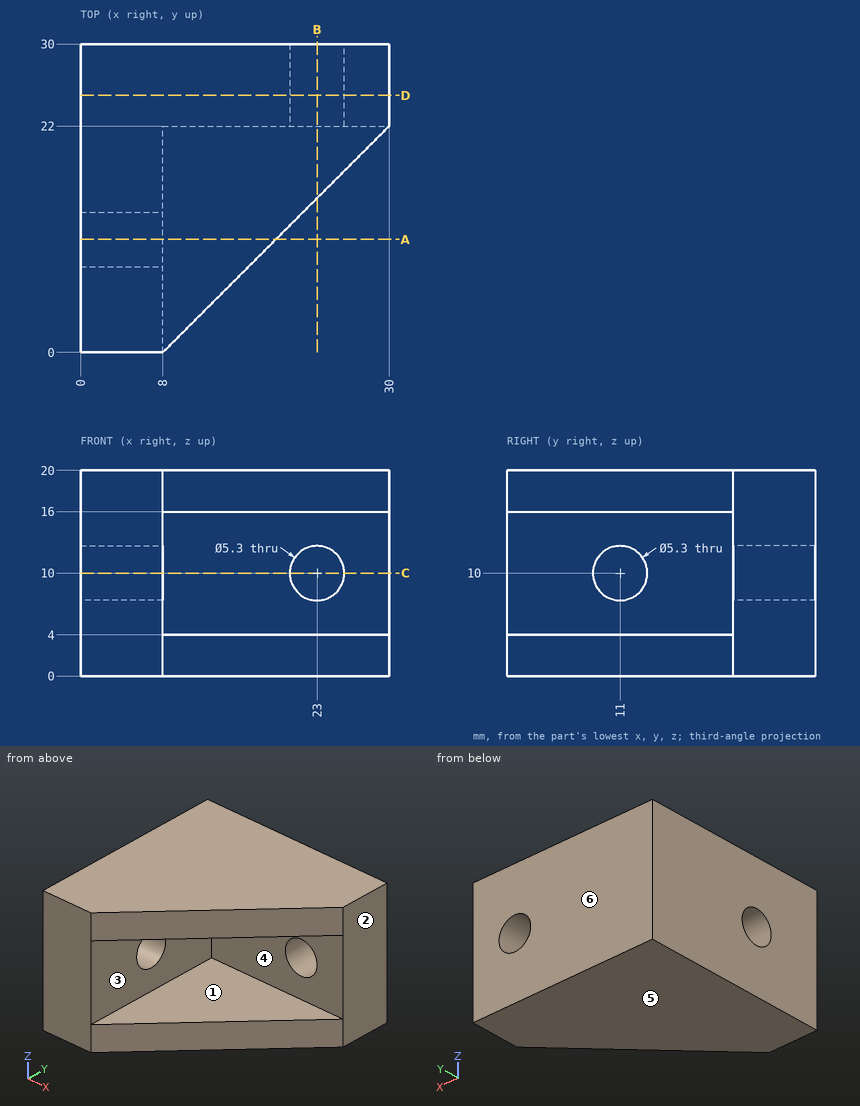
Answer from the drawing. Dimensions are ordinates in mm from the lowest x, y and z of the part. A direction names the side the tool comes from. Round coordinates to 2 decimals unless told otherwise and drop trailing zeros. Write each loop counter-clockwise with the first axis right and the second up, starting at its lowest first coordinate (ties: lowest second). Pieces come first, ordered by that corner, then holes. Notation, with made-up numbers: (39, 57) -> (81, 57) arc R18 cw to (81, 79) -> close; hole circle Ø5 at (18.25, -39). An arc over 180 degrees is marked (long way). Answer in a Markdown table with one row per item. Add a question column.
1) Given P1, Ø6, axis at y = 12, z = 7.5, coming from the -X side; P2, Ø5, axis at x = 23, z = 10, coming from the -Y side; P3, Ø1.5, axis at x = 11, z = 17, coming from the -Y side; P4, Ø1, axis at x = 11, z = 11, coming from the -Y side, each flat-ended and moving along its own axis, determine where each tip first touches the part or whether it passes through.
2) Determine the mould class of the marked faces 3, 4, 5 and 6 for opening direction Z: pulls with the +Z half, pulls with the -Z half, needs draft (parallel to the pull), parting line crosses it, or undercut.
3) Find section D-D, the plane y = 25. Determine the outline of the cut face in (x, z), and give its area (3 significant figures).
4) Find section B-B, the plane x = 23. Determine the outline of the cut face in (y, z), and give its area (3 significant figures).
5) Find section A-A, the plane y = 11. Determine the outline of the cut face in (x, z).
6) Consider line 1 (Z direction, x = 16.5, y = 12.5); line 2 (Z direction, x = 23, y = 24); line 3 (Y direction, x = 5.75, z = 10). Determine where each line is inside the solid, lowest interval first.
7) Find section C-C, the plane z = 10. Determine the outline of the cut face in (x, y).
8) Which of the six approach directions +Z, -Z, +X, -X, +Y, -Y give full straight-line access (tool end or side, diameter ignored) to the marked faces 1 and 2?
Findings below:
| question | item | result |
|---|---|---|
| 1 | P1 | x = 0 |
| 1 | P2 | through |
| 1 | P3 | y = 2.25 |
| 1 | P4 | y = 22 |
| 2 | face 3 | undercut |
| 2 | face 4 | undercut |
| 2 | face 5 | pulls with the -Z half |
| 2 | face 6 | needs draft |
| 3 | outline | (0, 0) -> (30, 0) -> (30, 20) -> (0, 20) -> close; hole circle Ø5.3 at (23, 10) |
| 3 | area | 578 mm² |
| 4 | outline | (15, 0) -> (30, 0) -> (30, 7.35) -> (22, 7.35) -> (22, 4) -> (15, 4) -> close; (15, 16) -> (22, 16) -> (22, 12.65) -> (30, 12.65) -> (30, 20) -> (15, 20) -> close |
| 4 | area | 174 mm² |
| 5 | outline | (0, 0) -> (19, 0) -> (19, 4) -> (8, 4) -> (8, 7.35) -> (0, 7.35) -> close; (0, 12.65) -> (8, 12.65) -> (8, 16) -> (19, 16) -> (19, 20) -> (0, 20) -> close |
| 6 | line 1 | 0 to 4, 16 to 20 |
| 6 | line 2 | 0 to 7.35, 12.65 to 20 |
| 6 | line 3 | 0 to 8.35, 13.65 to 30 |
| 7 | outline | (0, 0) -> (8, 0) -> (8, 8.35) -> (0, 8.35) -> close; (0, 13.65) -> (8, 13.65) -> (8, 22) -> (20.35, 22) -> (20.35, 30) -> (0, 30) -> close; (25.65, 22) -> (30, 22) -> (30, 30) -> (25.65, 30) -> close |
| 8 | face 1 | +X, -Y |
| 8 | face 2 | +Z, -Z, +X, +Y, -Y |
